Input: part model. Units: mm. Frame: model coordinates. A direction names the side the tool comes from. Coordinates: 2 decimals unless noted, no trailing zeros. Write each loop counter-clockwise with the first axis right and the second up, starting at its lowest first coordinate (ties: lowest second). Pieces come first, ordered by that corner, then holes. Notation, with made-up numbers: (-35, -19.5) - (-26, -19.5) arc R20 ccw to (-26, 0.5) - close; hole circle Ø10 at (23.25, -19.5). An arc over 180 degrees is marked (long way). Use a Markdown table: item, result. Add a question column.
Q1. Section query C-C (y = -41.5). Return the cut outline in (x, z).
Q2. Pin query (flat end, axial travel): P1, Ø1.5, axis at x = 0.5, y = -5, coming from the +Z side; P2, Ø1.5, axis at x = 2.5, y = -28.5, coming from the -Z side; P3, Ø1.6, axis at y = -14, z = 15, coming from the -X side; P4, Ø1.5, axis at y = 10, z = 33.19, coming from the +X side. Return the tip coordinate at first contact, or that it passes through.
Q3. Mould query, pull axis Z, two halves, no side actions, for faces 1 (the face through (2, -64, -64)), 2 (the face through (1, 15, -14)), 3 (the face through (1.48, 2.78, 15.27)). Classes: released by +Z, released by -Z, zero draft, split by the parting line, or undercut.
Q4. Set-up query: faces 4 (the face through (1, 5, -32)), 5 (the face through (1, 8.5, 15)), 6 (the face through (1, -66, -27)). Return all of +Z, -Z, +X, -X, +Y, -Y with unobstructed straight access to the full face (end or side cutting, diameter ignored); none if empty.
Q5. Section query B-B (z = -55). Return the cut outline in (x, y).
Q6. Section query D-D (z = 47). Return the cut outline in (x, y).
Q7. Section query A-A (z = -25). Return the cut outline in (x, y), then the cut area to 3 significant figures.
Q8. Material intervals for probe 1 along Y at (x, z) = (1.6, -25); probe 2 along Y at (x, z) = (1.5, 15) (3 decimals); probe 3 along Y at (x, z) = (0.95, 50), sorted ascending. Write a range as from..to.
from build123d import *

# Parameters (mm, degrees)
SKETCH1_R           = 15
SKETCH1_R_2         = 3
SKETCH1_R_3         = 1.25
SKETCH1_R_4         = 0.625
SKETCH1_W           = 10
SKETCH1_H           = 2.5
SKETCH1_W_2         = 16
SKETCH1_H_2         = 3.5
BOSS_EXTRUDE1_DEPTH = 3
FILLET1_R           = 5
FILLET2_R           = 1


with BuildPart() as part:
    # Sketch1 → Boss-Extrude1 (new body)
    with BuildSketch(Plane(origin=(0, 0, 0), x_dir=(0, 0, -1), z_dir=(1, 0, 0))):
        with BuildLine():
            Line((0, 5), (65, 5))
            Line((65, 5), (65, 15))
            Line((65, 15), (-35, 15))
            Line((-35, 15), (-65.988977704, -10.781451876))
            ThreePointArc((-65.988977704, -10.781451876), (-74.331609313, -35.742193679), (-55.709440186, -54.339315783))
            Line((-55.709440186, -54.339315783), (-6, -66))
            Line((-6, -66), (65, -66))
            Line((65, -66), (65, -54))
            Line((65, -54), (0, -54))
            Line((0, -54), (0, 5))
        make_face()
        with Locations((-50, -30)):
            Circle(SKETCH1_R, mode=Mode.SUBTRACT)
        with Locations((55, 10)):
            Circle(SKETCH1_R_2, mode=Mode.SUBTRACT)
        with Locations((25, 10)):
            Circle(SKETCH1_R_2, mode=Mode.SUBTRACT)
        with Locations((-33.192050804, 10)):
            Circle(SKETCH1_R_3, mode=Mode.SUBTRACT)
        with Locations((-50, -50)):
            Circle(SKETCH1_R_3, mode=Mode.SUBTRACT)
        with Locations((-70, -30)):
            Circle(SKETCH1_R_3, mode=Mode.SUBTRACT)
        with Locations((-10, -59.255419511)):
            Circle(SKETCH1_R_3, mode=Mode.SUBTRACT)
        with Locations((-25, 4)):
            Circle(SKETCH1_R_3, mode=Mode.SUBTRACT)
        with Locations((-15, 4)):
            Circle(SKETCH1_R_3, mode=Mode.SUBTRACT)
        with Locations((-15, -14)):
            Circle(SKETCH1_R_4, mode=Mode.SUBTRACT)
        with Locations((-21.5, -14)):
            Circle(SKETCH1_R_4, mode=Mode.SUBTRACT)
        with Locations((-15, 9.75)):
            Rectangle(SKETCH1_W, SKETCH1_H, mode=Mode.SUBTRACT)
        with Locations((53, -60)):
            Rectangle(SKETCH1_W_2, SKETCH1_H_2, mode=Mode.SUBTRACT)
    extrude(amount=BOSS_EXTRUDE1_DEPTH)

    # Fillet1
    fillet1_edges = [part.edges().sort_by_distance(p)[0] for p in [
        (1.5, -66, -65),
        (1.5, -66, 6),
        (1.5, 15, 35),
        (1.5, 15, -65),
    ]]
    fillet(fillet1_edges, radius=FILLET1_R)

    # Fillet2
    fillet2_edges = [part.edges().sort_by_distance(p)[0] for p in [
        (1.5, 5, -65),
        (1.5, -54, -65),
    ]]
    fillet(fillet2_edges, radius=FILLET2_R)


solid = part.part
Values follow:
| question | item | result |
|---|---|---|
| 1 | outline | (0, 0) - (3, 0) - (3, 40.37) - (0, 40.37) - close; (0, 59.63) - (3, 59.63) - (3, 72.2) - (0, 72.2) - close |
| 2 | P1 | z = 59.94 |
| 2 | P2 | z = 0 |
| 2 | P3 | x = 0 |
| 2 | P4 | through |
| 3 | face 1 | released by -Z |
| 3 | face 2 | zero draft |
| 3 | face 3 | undercut |
| 4 | face 4 | -Z, +X, -X |
| 4 | face 5 | +X, -X |
| 4 | face 6 | +Z, -Z, +X, -X, -Y |
| 5 | outline | (0, -66) - (3, -66) - (3, -61.75) - (0, -61.75) - close; (0, -58.25) - (3, -58.25) - (3, -54) - (0, -54) - close; (0, 5) - (3, 5) - (3, 7) - (0, 7) - close; (0, 13) - (3, 13) - (3, 15) - (0, 15) - close |
| 6 | outline | (0, -56.38) - (3, -56.38) - (3, -44.7) - (0, -44.7) - close; (0, -15.3) - (3, -15.3) - (3, 5.02) - (0, 5.02) - close |
| 7 | outline | (0, -66) - (3, -66) - (3, -54) - (0, -54) - close; (0, 5) - (3, 5) - (3, 7) - (0, 7) - close; (0, 13) - (3, 13) - (3, 15) - (0, 15) - close |
| 7 | area | 48.0 mm2 |
| 8 | probe 1 | -66..-54, 5..7, 13..15 |
| 8 | probe 2 | -63.889..-14.625, -13.375..2.75, 5.25..8.5, 11..15 |
| 8 | probe 3 | -55.68..-51.25, -48.75..-45, -15..2.52 |
